from build123d import *

# Parameters (mm, degrees)
BOSS_EXTRUDE1_DEPTH          = 3.175
F_3_8_CLEARANCE_HOLE2_D      = 10.0838
F_1_8_0_125_DIAMETER_HOLE1_D = 3.175


with BuildPart() as part:
    # Sketch1 → Boss-Extrude1 (new body)
    with BuildSketch(Plane.XY):
        with BuildLine():
            Line((-12.7, -23.8125), (-12.7, 23.8125))
            ThreePointArc((-12.7, 23.8125), (0, 36.5125), (12.7, 23.8125))
            Line((12.7, 23.8125), (12.7, -23.8125))
            ThreePointArc((12.7, -23.8125), (0, -36.5125), (-12.7, -23.8125))
        make_face()
    extrude(amount=BOSS_EXTRUDE1_DEPTH)

    # 3/8 Clearance Hole2 (through all)
    with Locations(Plane.XY.offset(3.175)):
        with Locations((0, 23.8125), (0, -23.8125)):
            Hole(F_3_8_CLEARANCE_HOLE2_D / 2)

    # 1/8 (0.125) Diameter Hole1 (through all)
    with Locations(Plane.XY.offset(3.175)):
        with Locations((6.35, -6.35), (6.35, 6.35), (-6.35, -6.35), (-6.35, 6.35)):
            Hole(F_1_8_0_125_DIAMETER_HOLE1_D / 2)


solid = part.part
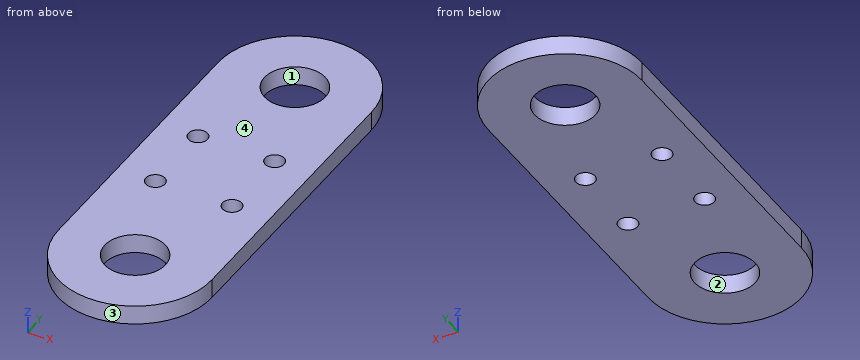
Geometry: final body of the model. Coordinates: model frame, mm. Face numbers are marked on the shaded views. Give positions to 0.01 mm unless a question says otherwise; leave off trailing zeros. Write each loop counter-clockwise with the first axis right and the second up, starting at its lowest first coordinate (ties: lowest second). Pieces come first, ordered by that corner, then holes.
(1) Cut plane D-D, the plane y = 23. Return loops of the section in (x, z) (3 decimals), then the cut area to 3 significant figures.
(2) First-contact query: P1, Ø1.5, axis at x = 10, z = 1.5, coming from the -Y side. Flat tip, straight axial feed; report the tip coordinate or a pass-through.
(3) Cut plane C-C, the plane z = 2.1. Give the number of separate pieces and of enclosed holes in the cut face, then the cut area to 3 significant figures.
(4) Ray query, line 1 (X direction, y = 6.5, z = 3); line 2 (Y direction, x = 0, z = 1.9); line 3 (Y direction, x = -5.75, z = 0.7). Return the intervals inside material, ascending.
(5) Mould query, pull axis X, two halves, no side actions, for the marked faces 1, 2, 3 and 4. Classes: released by +X, released by -X, zero draft, split by the parting line, or undercut.
(6) Cut plane A-A, the plane y = 6.35. Return loops of the section in (x, z) (1 decimal), then the cut area to 3 significant figures.
(7) Cut plane B-B, the plane x = 0. Return loops of the section in (y, z) (1 decimal), then the cut area to 3 significant figures.
Values follow:
1. outline: (-12.7, 0) - (-4.976, 0) - (-4.976, 3.175) - (-12.7, 3.175) - close; (4.976, 0) - (12.7, 0) - (12.7, 3.175) - (4.976, 3.175) - close
1. area: 49.0 mm2
2. P1: stops at y = -32.51
3. separate pieces: 1
3. enclosed holes: 6
3. area: 1,520 mm2
4. line 1: x = -12.7 to -7.93, -4.77 to 4.77, 7.93 to 12.7
4. line 2: y = -36.51 to -28.85, -18.77 to 18.77, 28.85 to 36.51
4. line 3: y = -35.14 to -7.82, -4.88 to 4.88, 7.82 to 35.14
5. face 1: undercut
5. face 2: undercut
5. face 3: split by the parting line
5. face 4: zero draft
6. outline: (-12.7, 0) - (-7.9, 0) - (-7.9, 3.2) - (-12.7, 3.2) - close; (-4.8, 0) - (4.8, 0) - (4.8, 3.2) - (-4.8, 3.2) - close; (7.9, 0) - (12.7, 0) - (12.7, 3.2) - (7.9, 3.2) - close
6. area: 60.5 mm2
7. outline: (-36.5, 0) - (-28.9, 0) - (-28.9, 3.2) - (-36.5, 3.2) - close; (-18.8, 0) - (18.8, 0) - (18.8, 3.2) - (-18.8, 3.2) - close; (28.9, 0) - (36.5, 0) - (36.5, 3.2) - (28.9, 3.2) - close
7. area: 168 mm2
